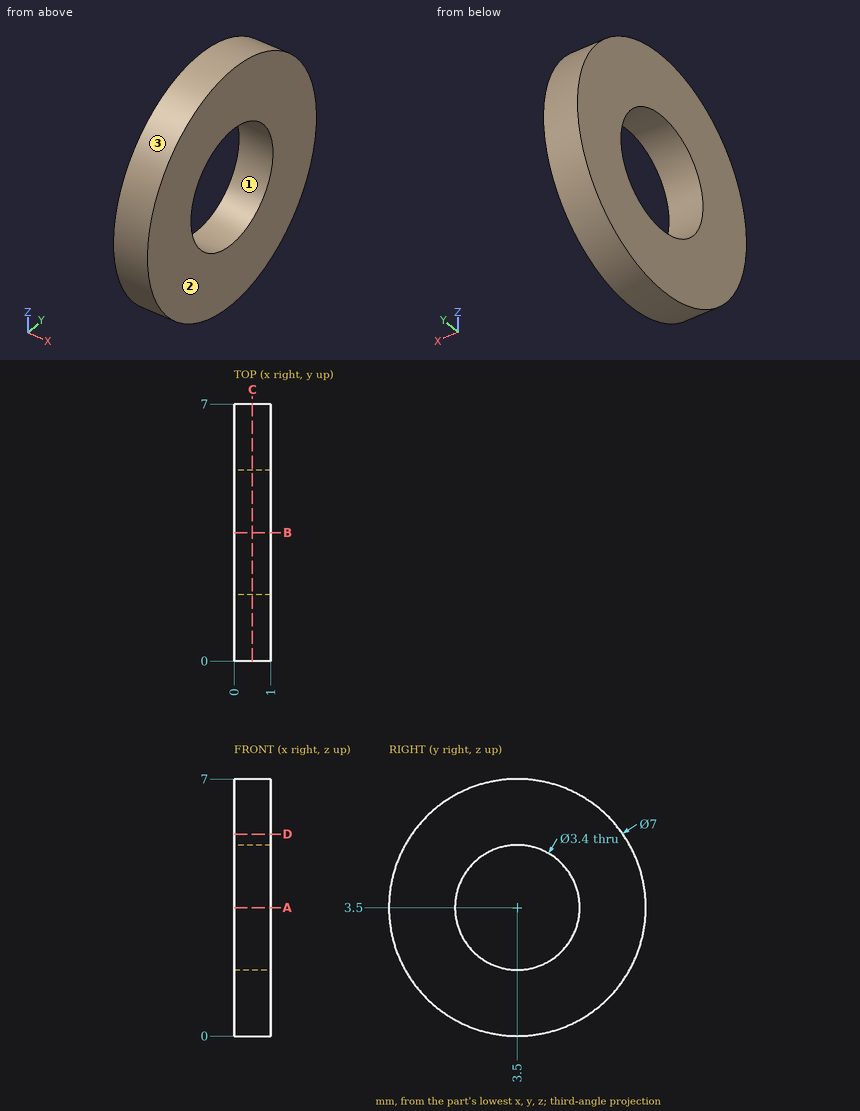
Can you work these out from the drawing? Everything is in mm from the part's minimum corner. Give positions to 0.01 mm unless a question says otherwise; leave off trailing zeros. Order: outer loops, then holes, each group sorted by start corner. A loop starts at its lowest first (then second) coordinate and runs counter-clockwise, first axis right, second up. Notation, with made-up numbers: M 43.5,66 L 85.5,66 A20 ccw 85.5,89 Z; hole C -16,17 d4. An arc over 180 degrees is marked long. One line per item, written item: value.
Item 1: For pin 1 (3 mm diameter, centred on y = 3.5, z = 3.5, fed in from -X), with a flat end and sliding along its axis, tell me the tip position at first contact or that it passes through.
Verdict:
pin 1: through
Item 2: If we mould it in two halves opening along Z, with no side actions, what happens to the marked faces 1, 2 and 3? For each: pulls with the +Z half, pulls with the -Z half, needs draft (parallel to the pull), parting line crosses it, or undercut.
Verdict:
face 1: undercut
face 2: needs draft
face 3: parting line crosses it
Item 3: If we section it at A-A on z = 3.5: Write out the boundary of the cut face in (x, y), and give its area (3 significant figures).
Verdict:
outline: M 0,0 L 1,0 L 1,1.8 L 0,1.8 Z; M 0,5.2 L 1,5.2 L 1,7 L 0,7 Z
area: 3.60 mm2
Item 4: If we section it at C-C on x = 0.5: Write out the boundary of the cut face in (y, z).
Verdict:
outline: C 3.5,3.5 d7; hole C 3.5,3.5 d3.4
Item 5: If we section it at D-D on z = 5.5: Write out the boundary of the cut face in (x, y).
Verdict:
outline: M 0,0.63 L 1,0.63 L 1,6.37 L 0,6.37 Z
Item 6: Please list where these lines run through material, in increasing order: line 1 (Y direction, x = 0.85, z = 3.5); line 2 (Y direction, x = 0.85, z = 3); line 3 (Z direction, x = 0.5, y = 3.25).
Verdict:
line 1: 0 to 1.8, 5.2 to 7
line 2: 0.04 to 1.88, 5.12 to 6.96
line 3: 0.01 to 1.82, 5.18 to 6.99
